Could you check a few things on this model? Use its own coordinates, in mm. Face numbers are marked on the shaded views. Give positions to 0.01 mm unless a question says otherwise; leave off trailing zeros. Order: outer loops, then holes, each group sorted by start corner. A loop starts at its lowest first (then second) coordinate and runs counter-clockwise, first axis right, second up.
(1) Imagine slicing it at C-C, the plane y = -2.5. Write out the boundary of the cut face in (x, z), then the cut area to 3 significant figures.
(2) Imagine slicing it at A-A, the plane z = -3.25. Write out the boundary of the cut face in (x, y).
(3) Will these pins go through, and if not, where does the flat tip stop? pin 1 (1.5 mm diameter, centred on x = -8, y = 0, fed in from +Z); pin 2 (8 mm diameter, centred on x = -11.5, z = -8.5, fed in from +Y).
(4) Imagine slicing it at B-B, the plane y = 11.25. Write out the boundary of the cut face in (x, z).
(5) Imagine slicing it at D-D, the plane x = 2. Write out the boundary of the cut face in (y, z), then the cut area to 3 significant figures.
(6) If we mould it in two halves opening along Y, with no side actions, what happens to the marked faces 1, 2, 3 and 4? For each: released by +Y, released by -Y, zero draft, split by the parting line, or undercut.
(7) If I drill on probe 1 along Z at (x, y) = (12, 9); probe 2 along Y at (x, z) = (0, 11); probe 3 along X at (y, z) = (10.5, 10), over which ranges is the centre line in solid material (lowest first)?
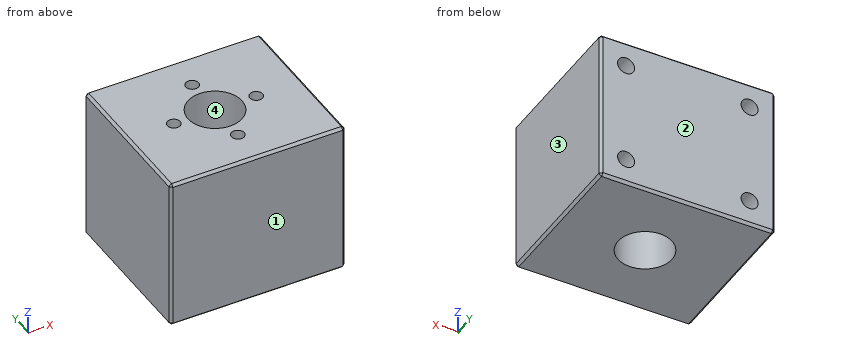
from build123d import *

# Parameters (mm, degrees)
SKETCH_1_W          = 34
SKETCH_1_H          = 30
EXTRUDE_1_DEPTH     = 15
SKETCH_3_R          = 5.25
CUT_EXTRUDE_1_DEPTH = 31
M3X0_5_1_D          = 2.5
M3X0_5_1_DEPTH      = 10
M3X0_5_1_TIP        = 0.751075774
M4X0_7_1_D          = 3.3
M4X0_7_1_DEPTH      = 20
M4X0_7_1_TIP        = 0.991420021
CHAMFER1_SIZE       = 0.5


with BuildPart() as part:
    # 草圖1 → 填料-伸長1 (new body, symmetric)
    with BuildSketch(Plane.XY):
        Rectangle(SKETCH_1_W, SKETCH_1_H)
    extrude(amount=EXTRUDE_1_DEPTH, both=True)

    # 草圖3 → 除料-伸長1 (cut, through all)
    with BuildSketch(Plane.XY.offset(15)):
        Circle(SKETCH_3_R)
    extrude(amount=-CUT_EXTRUDE_1_DEPTH, mode=Mode.SUBTRACT)

    # M3x0.5 螺紋孔1
    with Locations(Plane.XY.offset(15)):
        with Locations((8, 0), (-8, 0), (0, 8), (0, -8)):
            Hole(M3X0_5_1_D / 2, depth=M3X0_5_1_DEPTH)
            with Locations((0, 0, -(M3X0_5_1_DEPTH + M3X0_5_1_TIP / 2))):  # 118° drill point
                Cone(0, M3X0_5_1_D / 2, M3X0_5_1_TIP, mode=Mode.SUBTRACT)

    # M4x0.7 螺紋孔1
    with Locations(Plane(origin=(0, 15, 0), x_dir=(1, 0, 0), z_dir=(0, 1, 0))):
        with Locations((12, -10), (-12, 10), (-12, -10), (12, 10)):
            Hole(M4X0_7_1_D / 2, depth=M4X0_7_1_DEPTH)
            with Locations((0, 0, -(M4X0_7_1_DEPTH + M4X0_7_1_TIP / 2))):  # 118° drill point
                Cone(0, M4X0_7_1_D / 2, M4X0_7_1_TIP, mode=Mode.SUBTRACT)

    # Chamfer1
    chamfer1_edges = [part.edges().sort_by_distance(p)[0] for p in [
        (-17, 0, 15),
        (0, -15, 15),
        (17, 0, 15),
        (0, -15, -15),
        (-17, 0, -15),
        (0, 15, -15),
        (17, 0, -15),
        (0, 15, 15),
        (17, -15, 0),
        (-17, -15, 0),
        (-17, 15, 0),
        (17, 15, 0),
    ]]
    chamfer(chamfer1_edges, length=CHAMFER1_SIZE)


solid = part.part
Answer block:
1. outline: (-17, -14.5) - (-16.5, -15) - (-4.62, -15) - (-4.62, 15) - (-16.5, 15) - (-17, 14.5) - close; (4.62, -15) - (16.5, -15) - (17, -14.5) - (17, 14.5) - (16.5, 15) - (4.62, 15) - close; hole circle Ø3.3 at (-12, -10); hole circle Ø3.3 at (-12, 10); hole circle Ø3.3 at (12, -10); hole circle Ø3.3 at (12, 10)
1. area: 708 mm2
2. outline: (-17, -14.5) - (-16.5, -15) - (16.5, -15) - (17, -14.5) - (17, 14.5) - (16.5, 15) - (-16.5, 15) - (-17, 14.5) - close; hole circle Ø10.5 at (0, 0)
3. pin 1: stops at z = 4.7
3. pin 2: stops at y = 15
4. outline: (-17, -14.5) - (-16.5, -15) - (16.5, -15) - (17, -14.5) - (17, 14.5) - (16.5, 15) - (-16.5, 15) - (-17, 14.5) - close; hole circle Ø3.3 at (-12, -10); hole circle Ø3.3 at (-12, 10); hole circle Ø3.3 at (12, -10); hole circle Ø3.3 at (12, 10)
5. outline: (-15, -14.5) - (-14.5, -15) - (-4.85, -15) - (-4.85, 15) - (-14.5, 15) - (-15, 14.5) - close; (4.85, -15) - (14.5, -15) - (15, -14.5) - (15, 14.5) - (14.5, 15) - (4.85, 15) - close
5. area: 608 mm2
6. face 1: released by -Y
6. face 2: released by +Y
6. face 3: zero draft
6. face 4: undercut
7. probe 1: z = -15 to -11.65, -8.35 to 8.35, 11.65 to 15
7. probe 2: y = -15 to -9.25, -6.75 to -5.25, 5.25 to 6.75, 9.25 to 15
7. probe 3: x = -17 to -13.65, -10.35 to 10.35, 13.65 to 17
